```python
from build123d import *

# Parameters (mm, degrees)
BOSS_EXTRUDE1_DEPTH = 6
FILLET1_R           = 10
SKETCH2_R           = 2.5
CUT_EXTRUDE1_DEPTH  = 6
FILLET2_R           = 10
SKETCH5_R           = 1.25
CUT_EXTRUDE2_DEPTH  = 10
SKETCH6_R           = 1.25
CUT_EXTRUDE3_DEPTH  = 10
SKETCH7_R           = 1.65
CUT_EXTRUDE4_DEPTH  = 10
BOSS_EXTRUDE2_DEPTH = 6


with BuildPart() as part:
    # Sketch1 → Boss-Extrude1 (new body)
    with BuildSketch(Plane(origin=(0, 0, 0), x_dir=(1, 0, 0), z_dir=(0, 1, 0))):
        Polygon((21.213083016, -102.227633762), (35.213083016, -90.480238926), (35.213083016, -30.480238926), (21.213083016, -18.73284409), (21.213083016, 31.26715591), (35.213083016, 43.014550747), (35.213083016, 103.014550747), (-36.786916984, 103.014550747), (-36.786916984, 43.014550747), (-22.786916984, 31.26715591), (-22.786916984, -18.73284409), (-36.786916984, -30.480238926), (-36.786916984, -90.480238926), (-22.786916984, -102.227633762), align=None)
    extrude(amount=BOSS_EXTRUDE1_DEPTH)

    # Fillet1
    fillet1_edges = [part.edges().sort_by_distance(p)[0] for p in [
        (-22.786916984, 3, 102.227633762),
        (-36.786916984, 3, 90.480238926),
        (-36.786916984, 3, 30.480238926),
        (-22.786916984, 3, 18.73284409),
        (21.213083016, 3, 18.73284409),
        (35.213083016, 3, 30.480238926),
        (35.213083016, 3, 90.480238926),
        (21.213083016, 3, 102.227633762),
    ]]
    fillet(fillet1_edges, radius=FILLET1_R)

    # Sketch2 → Cut-Extrude1 (cut)
    with BuildSketch(Plane.XZ):
        with Locations(Location((-0.786916984, 60.480238926, 0), (0, 0, 270))):
            Circle(SKETCH2_R)
    extrude(amount=-CUT_EXTRUDE1_DEPTH, mode=Mode.SUBTRACT)

    # Fillet2
    fillet2_edges = [part.edges().sort_by_distance(p)[0] for p in [
        (-22.786916984, 3, -31.26715591),
        (-36.786916984, 3, -43.014550747),
        (35.213083016, 3, -43.014550747),
        (21.213083016, 3, -31.26715591),
    ]]
    fillet(fillet2_edges, radius=FILLET2_R)

    # Sketch5 → Cut-Extrude2 (cut)
    with BuildSketch(Plane(origin=(0, 6, 0), x_dir=(1, 0, 0), z_dir=(0, 1, 0))):
        with Locations(Location((15.213083016, 6.26715591, 0), (0, 0, 270))):
            Circle(SKETCH5_R)
        with Locations(Location((-16.786916984, 6.26715591, 0), (0, 0, 270))):
            Circle(SKETCH5_R)
    extrude(amount=-CUT_EXTRUDE2_DEPTH, mode=Mode.SUBTRACT)

    # Sketch6 → Cut-Extrude3 (cut)
    with BuildSketch(Plane.XZ):
        with Locations(Location((-22.567416075, 90.043344962, 0), (0, 0, 270))):
            Circle(SKETCH6_R)
        with Locations(Location((20.993582106, 90.043344962, 0), (0, 0, 270))):
            Circle(SKETCH6_R)
    extrude(amount=-CUT_EXTRUDE3_DEPTH, mode=Mode.SUBTRACT)

    # Sketch7 → Cut-Extrude4 (cut)
    with BuildSketch(Plane(origin=(0, 6, 0), x_dir=(1, 0, 0), z_dir=(0, 1, 0))):
        with Locations(Location((25.213083016, 73.014550747, 0), (0, 0, 270))):
            Circle(SKETCH7_R)
        with Locations(Location((-26.786916984, 73.014550747, 0), (0, 0, 270))):
            Circle(SKETCH7_R)
    extrude(amount=-CUT_EXTRUDE4_DEPTH, mode=Mode.SUBTRACT)

    # Sketch8 → Boss-Extrude2 (add)
    with BuildSketch(Plane(origin=(0, 6, 0), x_dir=(1, 0, 0), z_dir=(0, 1, 0))):
        with BuildLine():
            Line((-2.286916984, -57.882162715), (-2.286916984, -63.078315137))
            ThreePointArc((-2.286916984, -63.078315137), (-3.786916984, -60.480238926), (-2.286916984, -57.882162715))
        make_face()
        with BuildLine():
            Line((0.713083016, -57.882162715), (0.713083016, -63.078315137))
            ThreePointArc((0.713083016, -63.078315137), (2.213083016, -60.480238926), (0.713083016, -57.882162715))
        make_face()
    extrude(amount=-BOSS_EXTRUDE2_DEPTH)


solid = part.part
```
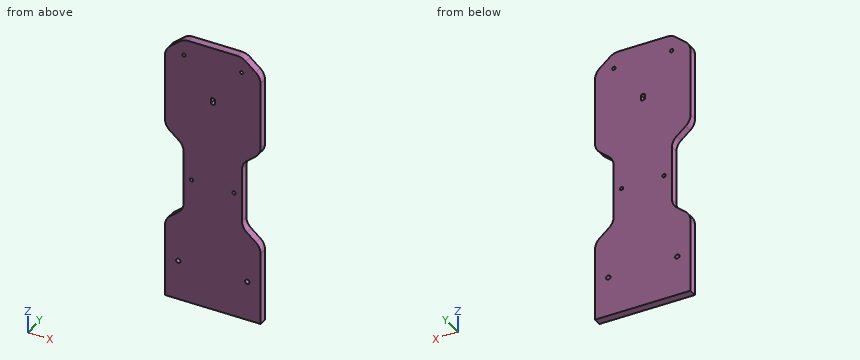
Model file for the job. Use its own axes, mm. Coordinates: 2 decimals unless noted, no trailing zeros. Loops run counter-clockwise (first coordinate to the right, second up) from the corner with the lowest first, then second, coordinate; pieces in that order, holes last. Notation, with made-up numbers: (-39, -8.5) -> (-28, -8.5) arc R24 cw to (-28, 12.5) -> close; hole circle Ø6 at (27.5, 69.5). An arc over 180 degrees is marked (long way). Answer as a JSON object with one key per item and string values.
Q1. Flat gauge pins, fed straight in: P1, Ø3, axis at x = -26.79, z = -73.01, coming from the -Y side; P2, Ø4, axis at x = -16.79, z = -6.27, coming from the -Y side; P3, Ø3, axis at y = 3, z = -2.5, coming from the -X side. Where does each tip first touch, or does it go through?
Report:
{"P1": "passes through", "P2": "stops at y = 0", "P3": "stops at x = -22.79"}
Q2. Cut at C-C (z = 25.5). List the corners of the cut face in (x, y).
Report:
{"outline": "(-30.85, 0) -> (29.28, 0) -> (29.28, 6) -> (-30.85, 6) -> close"}
Q3. Cut at B-B (y = 0.95). State how many separate pieces and enclosed holes the cut face has, and give its area (3 significant figures).
Report:
{"separate pieces": "1", "enclosed holes": "7", "area": "12,800 mm2"}
Q4. Cut at A-A (z = 1.5). List the corners of the cut face in (x, y).
Report:
{"outline": "(-22.79, 0) -> (21.21, 0) -> (21.21, 6) -> (-22.79, 6) -> close"}
Q5. Probe probe 1 along X at (y, z) = (2.1, 90); probe 2 along X at (y, z) = (4.75, 10); probe 3 along Z at (x, y) = (-33, 3). List the from-to ranges inside material, lowest first.
Report:
{"probe 1": "x = -35.87 to -23.82, -21.32 to 19.74, 22.24 to 34.3", "probe 2": "x = -22.79 to 21.21", "probe 3": "z = -103.01 to -39.84, 27.3 to 93.66"}
